Geometry: see drawing. Coordinates: mm, zero at the bounding-box minimum. Give positions to 0.01 mm unless a question says otherwise; leave off trailing zeros. Write each loop counter-clockwise with the first axis right and the second up, starting at its lowest first coordinate (ties: lowest second). Pieces come first, ordered by that corner, then holes. Notation, with made-up numbers: (78.25, 1.25) -> (137.25, 1.25) arc R23 ccw to (137.25, 16.25) -> close; hole circle Ø8 at (58, 83). An arc over 180 degrees is marked (long way). Use CSV: the item, a comma, the result in double quotes. Start each with the question number.
1) Section B-B (x = 105). Output: boundary loops of the cut face in (y, z).
2) Section A-A (z = 8.5). Output: boundary loops of the cut face in (x, y) (1 decimal).
3) Section C-C (y = 16.5). Output: boundary loops of the cut face in (x, z), plus the area to 3 significant figures.
4) Material intervals for line 1 (X direction, y = 21, z = 6.5) (1 decimal); line 2 (X direction, y = 26.5, z = 4.75) (1 decimal); line 3 (Y direction, x = 105.5, z = 8.5) (1 decimal), sorted ascending. Write a range as [from, to].
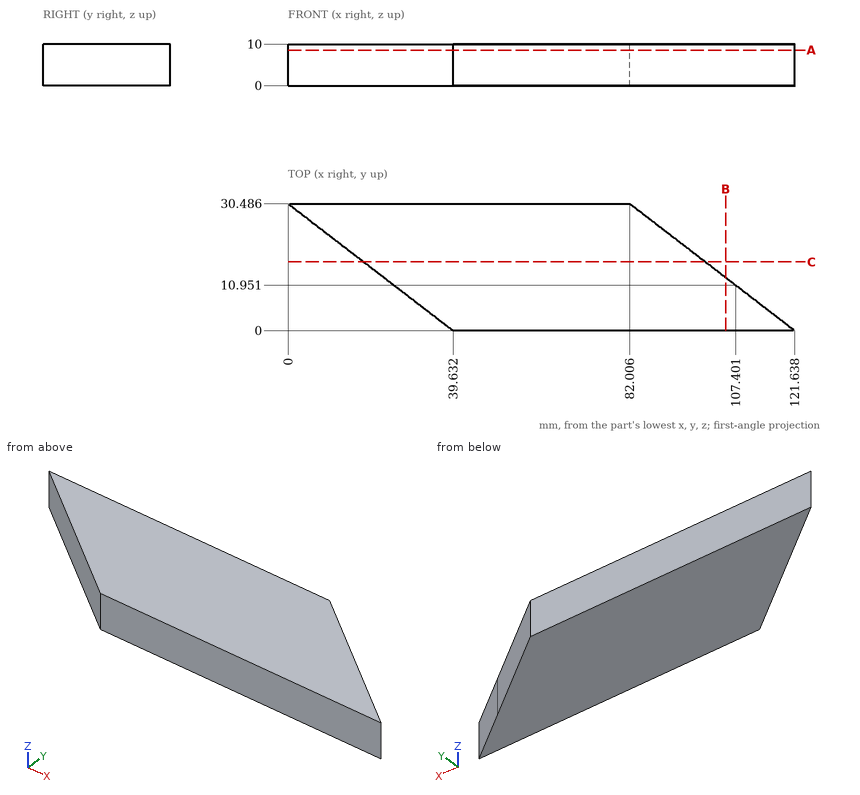
Answers follow:
1,outline,"(0, 0) -> (12.8, 0) -> (12.8, 10) -> (0, 10) -> close"
2,outline,"(0, 30.5) -> (39.6, 0) -> (121.6, 0) -> (107.4, 11) -> (82, 30.5) -> close"
3,outline,"(18.18, 0) -> (100.19, 0) -> (100.19, 10) -> (18.18, 10) -> close"
3,area,"820 mm^2"
4,line 1,"x = [12.3, 94.3]"
4,line 2,"x = [5.2, 87.2]"
4,line 3,"y = [0, 12.4]"
